from build123d import *

# Parameters (mm, degrees)
SKETCH1_R           = 55
BOSS_EXTRUDE1_DEPTH = 5
SKETCH2_R           = 6
SKETCH2_R_2         = 1.78
CUT_EXTRUDE1_DEPTH  = 5
SKETCH3_R           = 1.5
CUT_EXTRUDE2_DEPTH  = 5
CUT_EXTRUDE5_DEPTH  = 2.5
SKETCH6_R           = 1.8
CUT_EXTRUDE6_DEPTH  = 10
CUT_EXTRUDE7_DEPTH  = 3


with BuildPart() as part:
    # Sketch1 → Boss-Extrude1 (new body)
    with BuildSketch(Plane(origin=(0, 0, 0), x_dir=(1, 0, 0), z_dir=(0, 1, 0))):
        with Locations(Location((0, 0, 0), (0, 0, 270))):
            Circle(SKETCH1_R)
    extrude(amount=BOSS_EXTRUDE1_DEPTH)

    # Sketch2 → Cut-Extrude1 (cut)
    with BuildSketch(Plane(origin=(0, 5, 0), x_dir=(1, 0, 0), z_dir=(0, 1, 0))):
        with Locations(Location((0, 0, 0), (0, 0, 270))):
            Circle(SKETCH2_R)
        with Locations(Location((-13.47, -13.47, 0), (0, 0, 270))):
            Circle(SKETCH2_R_2)
        with Locations(Location((-13.47, 13.47, 0), (0, 0, 270))):
            Circle(SKETCH2_R_2)
        with Locations(Location((13.47, 13.47, 0), (0, 0, 270))):
            Circle(SKETCH2_R_2)
        with Locations(Location((13.47, -13.47, 0), (0, 0, 270))):
            Circle(SKETCH2_R_2)
    extrude(amount=-CUT_EXTRUDE1_DEPTH, mode=Mode.SUBTRACT)

    # Sketch3 → Cut-Extrude2 (cut)
    with BuildSketch(Plane(origin=(0, 5, 0), x_dir=(1, 0, 0), z_dir=(0, 1, 0))):
        with Locations(Location((4.5175, -7.824539523, 0), (0, 0, 270))):
            Circle(SKETCH3_R)
        with Locations(Location((-9.035, 0, 0), (0, 0, 270))):
            Circle(SKETCH3_R)
        with Locations(Location((4.5175, 7.824539523, 0), (0, 0, 270))):
            Circle(SKETCH3_R)
    extrude(amount=-CUT_EXTRUDE2_DEPTH, mode=Mode.SUBTRACT)

    # Sketch5 → Cut-Extrude5 (cut)
    with BuildSketch(Plane.XZ):
        Polygon((4.475281589, -11.519340051), (7.696181913, -9.708502003), (7.738400324, -6.013701476), (4.559718411, -4.129738996), (1.338818087, -5.940577043), (1.296599676, -9.635377571), align=None)
        Polygon((7.738400324, 9.635377571), (4.559718411, 11.519340051), (1.338818087, 9.708502003), (1.296599676, 6.013701476), (4.475281589, 4.129738996), (7.696181913, 5.940577043), align=None)
        Polygon((-12.213681913, 1.88396248), (-12.255900324, -1.810838048), (-9.077218411, -3.694800528), (-5.856318087, -1.88396248), (-5.814099676, 1.810838048), (-8.992781589, 3.694800528), align=None)
    extrude(amount=-CUT_EXTRUDE5_DEPTH, mode=Mode.SUBTRACT)

    # Sketch6 → Cut-Extrude6 (cut)
    with BuildSketch(Plane(origin=(0, 5, 0), x_dir=(1, 0, 0), z_dir=(0, 1, 0))):
        with Locations(Location((24.5, -5, 0), (0, 0, 270))):
            Circle(SKETCH6_R)
        with Locations(Location((-24.5, -5, 0), (0, 0, 270))):
            Circle(SKETCH6_R)
        with Locations(Location((-24.5, 5, 0), (0, 0, 270))):
            Circle(SKETCH6_R)
        with Locations(Location((24.5, 5, 0), (0, 0, 270))):
            Circle(SKETCH6_R)
    extrude(amount=-CUT_EXTRUDE6_DEPTH, mode=Mode.SUBTRACT)

    # Sketch7 → Cut-Extrude7 (cut)
    with BuildSketch(Plane(origin=(0, 0, 0), x_dir=(-1, 0, 0), z_dir=(0, -1, 0))):
        Polygon((26.809401077, -1), (22.190598923, -1), (19.881197846, -5), (22.190598923, -9), (26.809401077, -9), (29.118802154, -5), align=None)
        Polygon((-29.118802154, -5), (-26.809401077, -9), (-22.190598923, -9), (-19.881197846, -5), (-22.190598923, -1), (-26.809401077, -1), align=None)
        Polygon((26.809401077, 9), (22.190598923, 9), (19.881197846, 5), (22.190598923, 1), (26.809401077, 1), (29.118802154, 5), align=None)
        Polygon((-22.190598923, 9), (-26.809401077, 9), (-29.118802154, 5), (-26.809401077, 1), (-22.190598923, 1), (-19.881197846, 5), align=None)
    extrude(amount=-CUT_EXTRUDE7_DEPTH, mode=Mode.SUBTRACT)


solid = part.part
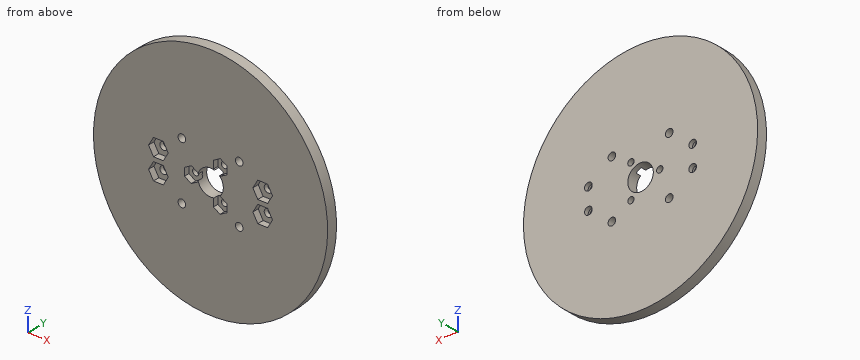
Can you work these out from the model? Positions are in its coordinate system, mm. Give positions to 0.01 mm unless a question says otherwise; leave off trailing zeros. Order: outer loops, then holes, each group sorted by start corner. A loop starts at its lowest first (then second) coordinate and runs counter-clockwise, first axis right, second up. Notation, with made-up numbers: M 48,13 L 54,13 A23 ccw 54,27 Z; hole C 48.5,9 d9. An arc over 180 degrees is marked long. Use a Markdown table: item, result. Add a question column.
Item 1: If I drill on L1, parallel to X at y = 3.1, z = 0 (3 decimals); L2, parallel to X at y = 0.45, z = 8; L3, parallel to X at y = 2.8, z = -13.47, over which ranges is the centre line in solid material (lowest first)? Write a range as [from, to].
Item 2: Suppose I cut it at D-D (z = -17). List the corners of the cut face in (x, y) for me, then the cut area to 3 significant figures.
Item 3: Suppose I cut it at B-B (x = 24.5). List the corners of the cut face in (y, z) for me.
Item 4: Suppose I cut it at A-A (y = 4.1). Count the separate pieces of the cut face and the enclosed holes in it, then the cut area to 3 significant figures.
Item 5: Suppose I cut it at C-C (z = 13.47). List the corners of the cut face in (x, y) for me, then the cut area to 3 significant figures.
Item 6: Will these pins go through, and if not, where does the flat tip stop? pin 1 (4 mm diameter, centred on x = 4.52, z = -7.82, fed in from -Y); pin 2 (1.5 mm diameter, centred on x = -24.5, y = 2, fed in from +Z); pin 3 (2 mm diameter, centred on y = 3.5, z = -19.5, fed in from -X).
Answer sheet:
| question | item | result |
|---|---|---|
| 1 | L1 | x = [-55, -10.535], [-7.535, -6], [6, 55] |
| 1 | L2 | x = [-54.42, -27.39], [-21.61, 1.32], [7.72, 21.61], [27.39, 54.42] |
| 1 | L3 | x = [-53.33, -15.25], [-11.69, 11.69], [15.25, 53.33] |
| 2 | outline | M -52.31,0 L 52.31,0 L 52.31,5 L -52.31,5 Z |
| 2 | area | 523 mm² |
| 3 | outline | M 0,-49.24 L 5,-49.24 L 5,-6.8 L 3,-6.8 L 3,-9 L 0,-9 Z; M 0,-1 L 3,-1 L 3,-3.2 L 5,-3.2 L 5,3.2 L 3,3.2 L 3,1 L 0,1 Z; M 0,9 L 3,9 L 3,6.8 L 5,6.8 L 5,49.24 L 0,49.24 Z |
| 4 | separate pieces | 1 |
| 4 | enclosed holes | 12 |
| 4 | area | 9,290 mm² |
| 5 | outline | M -53.33,0 L -15.25,0 L -15.25,5 L -53.33,5 Z; M -11.69,0 L 11.69,0 L 11.69,5 L -11.69,5 Z; M 15.25,0 L 53.33,0 L 53.33,5 L 15.25,5 Z |
| 5 | area | 498 mm² |
| 6 | pin 1 | stops at y = 2.5 |
| 6 | pin 2 | stops at z = 49.61 |
| 6 | pin 3 | stops at x = -51.8 |
